```python
from build123d import *

# Parameters (mm, degrees)
SKETCH1_W           = 100
SKETCH1_H           = 250
BOSS_EXTRUDE1_DEPTH = 1000
SKETCH2_R           = 45
BOSS_EXTRUDE2_DEPTH = 25
SKETCH3_R           = 10
CUT_EXTRUDE1_DEPTH  = 25


with BuildPart() as part:
    # Sketch1 → Boss-Extrude1 (new body)
    with BuildSketch(Plane(origin=(0, 0, 0), x_dir=(1, 0, 0), z_dir=(0, 1, 0))):
        Rectangle(SKETCH1_W, SKETCH1_H)
    extrude(amount=BOSS_EXTRUDE1_DEPTH)

    # Sketch2 → Boss-Extrude2 (add)
    with BuildSketch(Plane(origin=(50, 0, 0), x_dir=(0, 0, -1), z_dir=(1, 0, 0))):
        with Locations(Location((0, 925, 0), (0, 0, 180))):
            Circle(SKETCH2_R)
    extrude(amount=BOSS_EXTRUDE2_DEPTH)

    # Sketch3 → Cut-Extrude1 (cut)
    with BuildSketch(Plane(origin=(75, 0, 0), x_dir=(0, 0, -1), z_dir=(1, 0, 0))):
        with Locations((0, 925)):
            Circle(SKETCH3_R)
    extrude(amount=-CUT_EXTRUDE1_DEPTH, mode=Mode.SUBTRACT)


solid = part.part
```
For this review, take the finished solid that the model builds, in its own axes (mm). A direction names the side the tool comes from. Give positions to 0.01 mm unless a question says otherwise; leave off trailing zeros. Write each loop counter-clockwise with the first axis right and the second up, starting at its lowest first coordinate (ties: lowest second). Pieces come first, ordered by that corner, then holes. Notation, with made-up numbers: M 32.25,16.5 L 42.25,16.5 A22 ccw 42.25,38.5 Z; hole C -15.5,40.25 d2. An arc over 180 degrees is marked long. Answer as a JSON object with one key per item and string values. Group by question number.
Item 1: For pin 1 Ø10 at (y, z) = (426.5, 76.5) entering from +X, flat-tipped, find the tip position at first contact; note if it passes through.
Item 2: Consider section C-C on x = 63. Write out the cut boundary in (y, z), plus the area to 3 significant figures.
Item 3: Consider section A-A on y = 925. Write out the cut boundary in (x, z), plus the area to 4 significant figures.
Item 4: Draft analysis for pull direction Z (two halves, no side actions). For faces 3 (the cylindrical face through (62.675, 934.915, 1.302)), 4 (the flat face through (-1, 493, -125)), 5 (the flat face through (-1, 493, 125)), 6 (the flat face through (-1, 1000, -2)), state which applies: +Z half, -Z half, draft (parallel to the pull), parting line (faces both ways), or undercut.
Item 5: Consider section B-B on z = 0. Write out the cut boundary in (x, y).
Item 6: For probe 1 along Z at (x, y) = (61.25, 925); probe 2 along Y at (x, z) = (57.5, 0); probe 3 along X at (y, z) = (628, -10), list the stretches that pass through material, from the lowest coordinate up. Write a range as [from, to].
Item 7: Tool access review of faces 1 (the flat face through (-1, 0, -2)), 2 (the cylindrical face through (62.325, 887.056, 24.192)): name each direction out of +Z, -Z, +X, -X, +Y, -Y from which nothing blocks a thin tool from reaching the whole face with its end or side.
Item 8: Consider section D-D on y = 537. Write out the cut boundary in (x, z), plus the area to 3 significant figures.
Check result:
{
 "1": {"pin 1": "stops at x = 50"},
 "2": {"outline": "C 925,0 d90; hole C 925,0 d20", "area": "6,050 mm^2"},
 "3": {"outline": "M -50,-125 L 50,-125 L 50,-45 L 75,-45 L 75,-10 L 50,-10 L 50,10 L 75,10 L 75,45 L 50,45 L 50,125 L -50,125 Z", "area": "26,750 mm^2"},
 "4": {"face 3": "undercut", "face 4": "-Z half", "face 5": "+Z half", "face 6": "draft"},
 "5": {"outline": "M -50,0 L 50,0 L 50,880 L 75,880 L 75,915 L 50,915 L 50,935 L 75,935 L 75,970 L 50,970 L 50,1000 L -50,1000 Z"},
 "6": {"probe 1": "z = [-45, -10], [10, 45]", "probe 2": "y = [880, 915], [935, 970]", "probe 3": "x = [-50, 50]"},
 "7": {"face 1": "+Z, -Z, +X, -X, -Y", "face 2": "+X"},
 "8": {"outline": "M -50,-125 L 50,-125 L 50,125 L -50,125 Z", "area": "25,000 mm^2"}
}
